from build123d import *

# Parameters (mm, degrees)
F0_R     = 10
F1_DEPTH = 50
F2_R     = 10
F3_DEPTH = 50.001
F5_DEPTH = 35
F7_DEPTH = 27.501


with BuildPart() as f1:
    # F0 (on Top) → F1 (new body)
    with BuildSketch(Plane.XY):
        with BuildLine():
            Line((-60, 0), (0, 0))
            Line((0, 0), (0, 32))
            ThreePointArc((0, 32), (-15.646012, 51.520317), (-38.104279, 40.499123))
            ThreePointArc((-38.104279, 40.499123), (-52.271806, 26.921947), (-71.886688, 26.360722))
            ThreePointArc((-71.886688, 26.360722), (-96.772615, -0.721304), (-60, 0))
        make_face()
        with Locations((-20, 32)):
            Circle(F0_R, mode=Mode.SUBTRACT)
    extrude(amount=F1_DEPTH)

    # F2 (on face) → F3 (cut, through all)
    with BuildSketch(Plane.XY.offset(50)):
        with Locations((-78.540496, 7.5)):
            Circle(F2_R)
    extrude(amount=-F3_DEPTH, mode=Mode.SUBTRACT)

    # F4 (on face) → F5 (cut)
    with BuildSketch(Plane.XY.offset(50)):
        with BuildLine():
            ThreePointArc((-75.410873, 27.253619), (-66.093154, 23.15451), (-60, 15))
            Line((-60, 15), (0, 15))
            Line((0, 15), (0, 64.447676))
            Line((0, 64.447676), (-75.410873, 64.447676))
            Line((-75.410873, 64.447676), (-75.410873, 27.253619))
        make_face()
    extrude(amount=-F5_DEPTH, mode=Mode.SUBTRACT)

    # F6 (on face) → F7 (cut, through all)
    with BuildSketch(Plane(origin=(0, 15, 0), x_dir=(-1, 0, 0), z_dir=(0, 1, 0))):
        Polygon((0, 50), (0, 25), (50, 50), align=None)
    extrude(amount=-F7_DEPTH, mode=Mode.SUBTRACT)


solid = f1.part
Check sheet for the modelled part. Datum: model origin and axes. Units: mm. A direction names the side the tool comes from. Round coordinates to 2 decimals unless told otherwise and drop trailing zeros. Write each loop counter-clockwise with the first axis right and the second up, starting at its lowest first coordinate (ties: lowest second). Pieces come first, ordered by that corner, then holes. Notation, with made-up numbers: (53, 2.5) -> (109, 2.5) arc R9 cw to (109, 19.5) -> close; hole circle Ø3 at (-31, 34.5). An arc over 180 degrees is marked (long way). Answer as CSV lines item,"result". Start each with the question number.
1) Tool access check on faces 1 (the flat face through (-37, 15, 29)), 2 (the cylindrical face through (-52.013, 27.032, 7.395)), 3 (the flat face through (-30, 0, 19)). Record the directions out of +Z, -Z, +X, -X, +Y, -Y that give a thin tool (end or side, any length) a straight path to the whole face; none if there is none.
2) Go/stop test with flat-tipped pins: P1, Ø5, axis at x = -57, z = 24, coming from the +Y side; P2, Ø1.5, axis at y = 18, z = 33, coming from the +X side; P3, Ø16, axis at x = -78.54, y = 7.5, coming from the -Z side; P4, Ø8, axis at x = -17, z = 11.5, coming from the -Y side. Record where each tip stops, or that it passes through.
3) Release check for a two-part mould opening along X. For faces 4 (the flat face through (-24.65, 7.605, 37.325)), 5 (the cylindrical face through (-69, 10.5, 25.4)), 6 (the flat face through (-28.5, 25.5, 15)) record: pulls with the +X half, pulls with the -X half, needs draft (parallel to the pull), parting line crosses it, or undercut.
4) Section check C-C on y = 36. Enter the section's corners in (x, z).
5) Section check D-D on x = -74. Enter the section's corners in (y, z), and give its area (3 significant figures).
6) Section check A-A on x = -20. Enter the section's corners in (y, z).
7) Material ranges on line 1 (Y direction, x = -20, z = 7.5); line 2 (Z direction, x = -10, y = 36.5); line 3 (X direction, y = 32, z = 11.25), recorded low to high. Write a range as from..to.
8) Section check B-B on z = 32. Enter the section's corners in (x, y).
Found:
1,face 1,"+Z, +X, +Y"
1,face 2,"+Z, -Z, +Y"
1,face 3,"+Z, -Z, +X, -Y"
2,P1,"stops at y = 15"
2,P2,"stops at x = -61.08"
2,P3,"passes through"
2,P4,"stops at y = 0"
3,face 4,"pulls with the +X half"
3,face 5,"undercut"
3,face 6,"needs draft"
4,outline,"(-40.77, 0) -> (-29.17, 0) -> (-29.17, 15) -> (-40.77, 15) -> close; (-10.83, 0) -> (-0.4, 0) -> (-0.4, 15) -> (-10.83, 15) -> close"
5,outline,"(-11.98, 0) -> (-1.41, 0) -> (-1.41, 50) -> (-11.98, 50) -> close; (16.41, 0) -> (26.98, 0) -> (26.98, 50) -> (16.41, 50) -> close"
5,area,"1,060 mm^2"
6,outline,"(0, 0) -> (22, 0) -> (22, 15) -> (15, 15) -> (15, 35) -> (0, 35) -> close; (42, 0) -> (52, 0) -> (52, 15) -> (42, 15) -> close"
7,line 1,"y = 0..22, 42..52"
7,line 2,"z = 0..15"
7,line 3,"x = -44.34..-30, -10..0"
8,outline,"(-71.89, 26.36) arc R20 ccw (long way) to (-60, 0) -> (-14, 0) -> (-14, 15) -> (-60, 15) arc R20 ccw to start; hole circle Ø20 at (-78.54, 7.5)"
